The listing builds one solid part. Answer for the finished solid, in the listing's coordinates (mm). A direction names the side the tool comes from. Coordinates: 2 decimals unless noted, no trailing zeros. Order: outer loops, then holes, each group sorted by start corner. A loop starts at its lowest first (then second) coordinate and runs counter-clockwise, first axis right, second up.
from build123d import *

# Parameters (mm, degrees)
F0_R     = 1.25
F1_DEPTH = 2
F2_W     = 38
F2_H     = 42
F3_DEPTH = 2
F4_W     = 1.5
F4_H     = 4
F5_DEPTH = 6
F6_W     = 38
F6_H     = 4
F7_DEPTH = 8
F8_R     = 1.25
F9_DEPTH = 25


with BuildPart() as f1:
    # F0 (on Top) → F1 (new body)
    with BuildSketch(Plane.XY):
        Polygon((19, 19), (-19, 19), (-19, -23), (10, -23), (12, -23), (19, -23), align=None)
        with BuildLine():
            ThreePointArc((-14, -15.25), (-15.25, -14), (-14, -12.75))
            Line((-14, -12.75), (-14, 0))
            Line((-14, 0), (2, 0))
            Line((2, 0), (2, -15.25))
            Line((2, -15.25), (-14, -15.25))
        make_face(mode=Mode.SUBTRACT)
        with Locations((14, -14)):
            Circle(F0_R, mode=Mode.SUBTRACT)
        with Locations((-14, 14)):
            Circle(F0_R, mode=Mode.SUBTRACT)
        with Locations((14, 14)):
            Circle(F0_R, mode=Mode.SUBTRACT)
    extrude(amount=F1_DEPTH)

    # F2 (on face) → F3 (join)
    with BuildSketch(Plane.XY.offset(2)):
        with Locations((0, -2)):
            Rectangle(F2_W, F2_H)
        Polygon((2, -15.25), (-12.1236116251, -15.25), (-12.7009618943, -16.25), (-15.2990381057, -16.25), (-16.5980762114, -14), (-15.2990381057, -11.75), (-14, -11.75), (-14, 0), (2, 0), align=None, mode=Mode.SUBTRACT)
        Polygon((15.2990381057, -11.75), (16.5980762114, -14), (15.2990381057, -16.25), (12.7009618943, -16.25), (11.4019237886, -14), (12.7009618943, -11.75), align=None, mode=Mode.SUBTRACT)
        Polygon((-12.7009618943, 16.25), (-11.4019237886, 14), (-12.7009618943, 11.75), (-15.2990381057, 11.75), (-16.5980762114, 14), (-15.2990381057, 16.25), align=None, mode=Mode.SUBTRACT)
        Polygon((15.2990381057, 16.25), (16.5980762114, 14), (15.2990381057, 11.75), (12.7009618943, 11.75), (11.4019237886, 14), (12.7009618943, 16.25), align=None, mode=Mode.SUBTRACT)
    extrude(amount=F3_DEPTH)

    # F4 (on Top) → F5 (join)
    with BuildSketch(Plane.XY):
        with Locations((-9, -25)):
            Rectangle(F4_W, F4_H)
        with Locations((9, -25)):
            Rectangle(F4_W, F4_H)
    extrude(amount=F5_DEPTH)

    # F6 (on face) → F7 (join)
    with BuildSketch(Plane.XY.offset(4)):
        with Locations((0, -21)):
            Rectangle(F6_W, F6_H)
    extrude(amount=F7_DEPTH)

    # F8 (on face) → F9 (cut)
    with BuildSketch(Plane.XZ.offset(23)):
        with Locations((-9, 9)):
            Circle(F8_R)
        with Locations((9, 9)):
            Circle(F8_R)
    extrude(amount=-F9_DEPTH, mode=Mode.SUBTRACT)


solid = f1.part
1) Section D-D (x = 14) is taken. Give the vertices of the cut face in (y, z), then the cut area to 3 significant figures.
2) Determine the mould class of faces 5 (the face through (-0.3, 0.3, 4)), 6 (the face through (-19, -7, 3)), 7 (the face through (0, -23, 6)), 8 (the face through (-12.06, 15.14, 2.99)) for opening direction X: released by +X, released by -X, zero draft, split by the parting line, or undercut.
3) Section C-C (y = -8.5) is taken. Give the vertices of the cut face in (x, z).
4) Section A-A (x = 9) is taken. Give the vertices of the cut face in (y, z).
5) Consider L1, parallel to Y at x = -1, z = 0.5; L2, parallel to X at y = -11.5, z = 1.5; L3, parallel to Z at x = 9, y = -19.8. Determine where each line is inside the solid, lowest interval first.
6) Section B-B (z = 9) is taken. Give the vertices of the cut face in (x, y), then the cut area to 3 significant figures.
7) Each of these flat-tipped pins is pushed along its axis until it touches: P1, Ø1.2, axis at y = -26, z = 4, coming from the -X side; P2, Ø3, axis at x = 14, y = -14, coming from the +Z side; P3, Ø1, axis at x = -13.5, z = 2.5, coming from the -Y side; P4, Ø3, axis at y = -15.5, z = 6, coming from the -X side. Where does it stop, or does it pass through?
8) A tool of negligible diameter and unlimited length cuts with its end or side. For faces 1 (the face through (-8.25, -25, 3)), 2 (the face through (-14, 16.25, 3)), 3 (the face through (-15.25, -14.03, 0.99)), 4 (the face through (9, -25, 6)), from which of +Z, -Z, +X, -X, +Y, -Y can it reach the whole face along a straight path? Write none if from no direction.
Filled sheet:
1. outline: (-23, 0) - (-15.25, 0) - (-15.25, 2) - (-16.25, 2) - (-16.25, 4) - (-19, 4) - (-19, 12) - (-23, 12) - close; (-12.75, 0) - (12.75, 0) - (12.75, 2) - (11.75, 2) - (11.75, 4) - (-11.75, 4) - (-11.75, 2) - (-12.75, 2) - close; (15.25, 0) - (19, 0) - (19, 4) - (16.25, 4) - (16.25, 2) - (15.25, 2) - close
1. area: 172 mm2
2. face 5: zero draft
2. face 6: released by -X
2. face 7: undercut
2. face 8: undercut
3. outline: (-19, 0) - (-14, 0) - (-14, 4) - (-19, 4) - close; (2, 0) - (19, 0) - (19, 4) - (2, 4) - close
4. outline: (-27, 0) - (19, 0) - (19, 4) - (-19, 4) - (-19, 7.75) - (-23, 7.75) - (-23, 6) - (-27, 6) - close; (-23, 10.25) - (-19, 10.25) - (-19, 12) - (-23, 12) - close
5. L1: y = -23 to -15.25, 0 to 19
5. L2: x = -19 to -14, 2 to 19
5. L3: z = 0 to 7.75, 10.25 to 12
6. outline: (-19, -23) - (-10.25, -23) - (-10.25, -19) - (-19, -19) - close; (-7.75, -23) - (7.75, -23) - (7.75, -19) - (-7.75, -19) - close; (10.25, -23) - (19, -23) - (19, -19) - (10.25, -19) - close
6. area: 132 mm2
7. P1: stops at x = -9.75
7. P2: stops at z = 2
7. P3: stops at y = -23
7. P4: passes through
8. face 1: +Z, -Z, -Y
8. face 2: +Z
8. face 3: +Z, -Z
8. face 4: +Z, +X, -X, -Y
